Could you check a few things on this model? Use its own coordinates, in mm. A direction names the side the tool comes from. Give positions to 0.01 mm unless a question says otherwise; leave off trailing zeros. Write each loop counter-clockwise with the first axis right and the second up, starting at its lowest first coordinate (ties: lowest second). Pieces come first, ordered by that corner, then holes. Notation, with made-up numbers: M 74,30 L 98,30 A32 cw 98,66 Z; hole C -38.75,1 d6. An arc over 180 degrees is marked long. One line per item, written item: value.
```python
from build123d import *

# Parameters (mm, degrees)
SKETCH2_W           = 50
SKETCH2_H           = 50
BOSS_EXTRUDE1_DEPTH = 50
SKETCH4_W           = 40
SKETCH4_H           = 40
CUT_EXTRUDE1_DEPTH  = 50
SKETCH7_W           = 40
SKETCH7_H           = 40
CUT_EXTRUDE2_DEPTH  = 50
SKETCH10_W          = 45.5
SKETCH10_H          = 45.5
SKETCH10_W_2        = 41.063521317
SKETCH10_H_2        = 40.909775363
CUT_EXTRUDE3_DEPTH  = 2.5


with BuildPart() as part:
    # Sketch2 → Boss-Extrude1 (new body)
    with BuildSketch(Plane.XY):
        with Locations((25, 25)):
            Rectangle(SKETCH2_W, SKETCH2_H)
    extrude(amount=BOSS_EXTRUDE1_DEPTH)

    # Sketch4 → Cut-Extrude1 (cut)
    with BuildSketch(Plane.XY.offset(50)):
        with Locations((25, 25)):
            Rectangle(SKETCH4_W, SKETCH4_H)
    extrude(amount=-CUT_EXTRUDE1_DEPTH, mode=Mode.SUBTRACT)

    # Sketch7 → Cut-Extrude2 (cut)
    with BuildSketch(Plane(origin=(0, 0, 0), x_dir=(0, 0, -1), z_dir=(1, 0, 0))):
        with Locations((-25, 25)):
            Rectangle(SKETCH7_W, SKETCH7_H)
    extrude(amount=CUT_EXTRUDE2_DEPTH, mode=Mode.SUBTRACT)

    # Sketch10 → Cut-Extrude3 (cut)
    with BuildSketch(Plane(origin=(0, 0, 0), x_dir=(1, 0, 0), z_dir=(0, 1, 0))):
        with Locations((25, -25)):
            Rectangle(SKETCH10_W, SKETCH10_H)
        with Locations((25.031760659, -24.954887682)):
            Rectangle(SKETCH10_W_2, SKETCH10_H_2, mode=Mode.SUBTRACT)
    extrude(amount=CUT_EXTRUDE3_DEPTH, mode=Mode.SUBTRACT)


solid = part.part
```
1) I'm going to push a flat-ended pin straight in: pin 1 (2 mm diameter, centred on x = 29.5, y = 1.5, fed in from -Z). Where does the tip first touch, or does it pass through?
Outcome:
pin 1: stops at z = 0
2) If we section it at A-A, the plane z = 25: Write out the boundary of the cut face in (x, y), then the cut area to 3 significant figures.
Outcome:
outline: M 0,0 L 2.25,0 L 2.25,2.5 L 4.5,2.5 L 4.5,0 L 45.56,0 L 45.56,2.5 L 47.75,2.5 L 47.75,0 L 50,0 L 50,5 L 0,5 Z; M 0,45 L 50,45 L 50,50 L 0,50 Z
area: 489 mm^2
3) Please list where these lines run through material, in increasing order: L1, parallel to Y at x = 34.5, z = 14; L2, parallel to Y at x = 12, z = 3. Write a range as from..to.
Outcome:
L1: y = 0..5, 45..50
L2: y = 2.5..5, 45..50
4) If we section it at B-B, the plane y = 37.5: Write out the boundary of the cut face in (x, z).
Outcome:
outline: M 0,0 L 5,0 L 5,5 L 0,5 Z; M 0,45 L 5,45 L 5,50 L 0,50 Z; M 45,0 L 50,0 L 50,5 L 45,5 Z; M 45,45 L 50,45 L 50,50 L 45,50 Z
5) We'd pull the mould along X, two halves only. Please class faces 1 (the face through (45.564, 1, 25)), 2 (the face through (47, 25, 45)), 3 (the face through (50, 47, 25)): pulls with the +X half, pulls with the -X half, needs draft (parallel to the pull), parting line crosses it, or undercut.
Outcome:
face 1: undercut
face 2: needs draft
face 3: pulls with the +X half
6) If we section it at C-C, the plane x = 8.5: Write out the boundary of the cut face in (y, z).
Outcome:
outline: M 0,0 L 5,0 L 5,50 L 0,50 L 0,47.75 L 2.5,47.75 L 2.5,45.41 L 0,45.41 L 0,4.5 L 2.5,4.5 L 2.5,2.25 L 0,2.25 Z; M 45,0 L 50,0 L 50,50 L 45,50 Z
7) On a 3-axis mill with a long thin cutter (end or side, diameter ignored), from which of +Z, -Z, +X, -X, +Y, -Y can I reach the whole of each face in a straight line? I mean faces 4 (the face through (2, 25, 45)), 5 (the face through (25, 1, 2.25)), 6 (the face through (47, 25, 50)), 7 (the face through (25, 0, 25)), 8 (the face through (5, 25, 3)). Say none if no direction works.
Outcome:
face 4: +X, -X
face 5: -Y
face 6: +Z, +X, -X, +Y, -Y
face 7: +Z, -Z, +X, -X, -Y
face 8: +Z, -Z
